from build123d import *

# Parameters (mm, degrees)
SKETCH1_R               = 10.16
BOSS_EXTRUDE1_DEPTH     = 0.762
SKETCH2_R               = 8.636
BOSS_EXTRUDE2_DEPTH     = 6.096
SKETCH3_R               = 11.43
BOSS_EXTRUDE3_DEPTH     = 5.334
SKETCH4_R               = 3.2385
CUT_EXTRUDE1_DEPTH      = 25.654
SKETCH5_W               = 6.096
SKETCH5_H               = 1.016
CUT_EXTRUDE2_DEPTH      = 1.016
CIRPATTERN1_COUNT       = 22
SKETCH6_R               = 1.143
CUT_EXTRUDE3_DEPTH      = 22.098
CUT_EXTRUDE3_DEPTH_BACK = 22.098


with BuildPart() as part:
    # Sketch1 → Boss-Extrude1 (new body)
    with BuildSketch(Plane.XY):
        Circle(SKETCH1_R)
    extrude(amount=-BOSS_EXTRUDE1_DEPTH)

    # Sketch2 → Boss-Extrude2 (add)
    with BuildSketch(Plane(origin=(0, 0, -0.762), x_dir=(-1, 0, 0), z_dir=(0, 0, -1))):
        Circle(SKETCH2_R)
    extrude(amount=BOSS_EXTRUDE2_DEPTH)

    # Sketch3 → Boss-Extrude3 (add)
    with BuildSketch(Plane(origin=(0, 0, -6.858), x_dir=(-1, 0, 0), z_dir=(0, 0, -1))):
        Circle(SKETCH3_R)
    extrude(amount=BOSS_EXTRUDE3_DEPTH)

    # Sketch4 → Cut-Extrude1 (cut)
    with BuildSketch(Plane.XY):
        Circle(SKETCH4_R)
    extrude(amount=-CUT_EXTRUDE1_DEPTH, mode=Mode.SUBTRACT)

    # Sketch5 → Cut-Extrude2 (cut)
    with BuildSketch(Plane.ZY.offset(8.636)):
        with Locations((-3.81, 0)):
            Rectangle(SKETCH5_W, SKETCH5_H)
    cut_extrude2 = extrude(amount=-CUT_EXTRUDE2_DEPTH, mode=Mode.SUBTRACT)

    # CirPattern1: Cut-Extrude2 ×22 about axis
    cirpattern1_axis = Axis((0, 0, 0), (0, 0, 1))
    for i in range(1, CIRPATTERN1_COUNT):
        add(cut_extrude2.rotate(cirpattern1_axis, i * 360 / CIRPATTERN1_COUNT), mode=Mode.SUBTRACT)

    # Sketch6 → Cut-Extrude3 (cut, two sides)
    with BuildSketch(Plane(origin=(0, 0, 0), x_dir=(1, 0, 0), z_dir=(0, 1, 0))) as cut_extrude3_sk:
        with Locations((0, 9.652)):
            Circle(SKETCH6_R)
    extrude(amount=CUT_EXTRUDE3_DEPTH, mode=Mode.SUBTRACT)
    extrude(cut_extrude3_sk.sketch, amount=-CUT_EXTRUDE3_DEPTH_BACK, mode=Mode.SUBTRACT)


solid = part.part
Could you check a few things on this model? Use its own coordinates, in mm. A direction names the side the tool comes from. Round coordinates to 2 decimals unless told otherwise and drop trailing zeros. Order: outer loops, then holes, each group sorted by start corner. A loop starts at its lowest first (then second) coordinate and runs counter-clockwise, first axis right, second up.
(1) Imagine slicing it at A-A (x = 0). Write out the boundary of the cut face in (y, z) (1 decimal), plus the area to 3 significant figures.
Response values:
outline: (-11.4, -12.2) - (-3.2, -12.2) - (-3.2, -10.8) - (-11.4, -10.8) - close; (-11.4, -8.5) - (-3.2, -8.5) - (-3.2, 0) - (-10.2, 0) - (-10.2, -0.8) - (-8.6, -0.8) - (-8.6, -6.9) - (-11.4, -6.9) - close; (3.2, -12.2) - (11.4, -12.2) - (11.4, -10.8) - (3.2, -10.8) - close; (3.2, -8.5) - (11.4, -8.5) - (11.4, -6.9) - (8.6, -6.9) - (8.6, -0.8) - (10.2, -0.8) - (10.2, 0) - (3.2, 0) - close
area: 126 mm2
(2) Please list where these lines run through material, in increasing order: line 1 along Z through (x, y) = (0, 5) (3 decimals); line 2 along Z through (x, y) = (5.5, 6.25); line 3 along X through (y, z) = (-5.75, -3.5).
Response values:
line 1: z = -12.192 to -10.795, -8.509 to 0
line 2: z = -12.19 to -6.86, -0.76 to 0
line 3: x = -6.44 to -5.65, -5 to 5, 5.65 to 6.44
(3) Imagine slicing it at D-D (y = 9). Write out the boundary of the cut face in (x, z).
Response values:
outline: (-7.05, -12.19) - (7.05, -12.19) - (7.05, -6.86) - (-7.05, -6.86) - close; (-4.71, -0.76) - (4.71, -0.76) - (4.71, 0) - (-4.71, 0) - close; hole circle Ø2.29 at (0, -9.65)
(4) I'm going to push flat-ended pins straight in: pin 1 (0.5 mm diameter, centred on x = 8, z = -3, fed in from +Y); pin 2 (1.4 mm diameter, centred on x = 0, z = -9.652, fed in from -Y); pin 3 (4 mm diameter, centred on y = 3.5, z = -7.5, fed in from -X); pin 4 (0.5 mm diameter, centred on x = 8, z = -5, fed in from -Y). Where does each tip first touch, or does it pass through?
Response values:
pin 1: stops at y = 3.81
pin 2: passes through
pin 3: stops at x = -11.33
pin 4: stops at y = -3.81
(5) Which directions (+Z, -Z, +X, -X, +Y, -Y) give clear straight access to the entire face, cutting with the end or side of a thin tool? Please do faces 1 (the flat face through (-1.66, 7.97, -3.85)), 2 (the cylindrical face through (8.55, -1.22, -3.77)), 3 (the flat face through (6.56, 4.82, -3.85)), 4 (the flat face through (0.654, 8.117, -3.853)), 5 (the flat face through (-8, 0.508, -4)).
Response values:
face 1: +Y
face 2: +X, -Y
face 3: +X
face 4: none
face 5: -X
(6) Imagine slicing it at C-C (y = 0). Write out the boundary of the cut face in (x, z).
Response values:
outline: (-11.43, -12.19) - (-3.24, -12.19) - (-3.24, 0) - (-10.16, 0) - (-10.16, -0.76) - (-7.62, -0.76) - (-7.62, -6.86) - (-11.43, -6.86) - close; (3.24, -12.19) - (11.43, -12.19) - (11.43, -6.86) - (7.62, -6.86) - (7.62, -0.76) - (10.16, -0.76) - (10.16, 0) - (3.24, 0) - close
(7) Imagine slicing it at B-B (y = -9.5). Write out the boundary of the cut face in (x, z), plus the area to 3 significant figures.
Response values:
outline: (-6.36, -12.19) - (6.36, -12.19) - (6.36, -6.86) - (-6.36, -6.86) - close; (-3.6, -0.76) - (3.6, -0.76) - (3.6, 0) - (-3.6, 0) - close; hole circle Ø2.29 at (0, -9.65)
area: 69.2 mm2
